Model file for the job. Use its own axes, mm. A direction names the side the tool comes from. Coordinates: 2 decimals unless noted, no trailing zeros. Write each loop counter-clockwise with the first axis right and the second up, starting at its lowest first coordinate (ties: lowest second). Pieces come first, ordered by that corner, then holes. Notation, with made-up numbers: (20, 65.25) -> (51, 65.25) arc R32 ccw to (51, 91.25) -> close; hole circle Ø1 at (16.25, 40.25). An arc over 180 degrees is marked (long way). Answer as a JSON object with one key per item and string values. Group by question number.
Autodesk Inventor part; units mm, degrees
ref_plane "YZ Plane" through (0, 0, 0) normal (1, 0, 0) x (0, 1, 0)
ref_plane "XZ Plane" through (0, 0, 0) normal (0, 1, 0) x (-1, 0, 0)
ref_plane "XY Plane" through (0, 0, 0) normal (0, 0, 1) x (1, 0, 0)
sketch "Sketch1" plane through (0, 0, 0) normal (0, 1, 0) x (-1, 0, 0)
  circle A0 centre (0, 0) radius 87.5
  dimension "d0" = 175
extrude "Plate1" add sketch "Sketch1" along normal blind 4
sketch "Sketch2" plane through (0, 4, 0) normal (0, 1, 0) x (1, 0, 0)
  circle A0 centre (0, 0) radius 87.5
  arc A1 (73.3682, -12.9368) -> (73.3682, 12.9368) centre (0, 0) ccw construction
  arc A2 (79.7694, -14.0655) -> (79.7694, 14.0655) centre (0, 0) ccw
  arc A3 (66.9669, -11.8081) -> (66.9669, 11.8081) centre (0, 0) ccw
  arc A4 (66.9669, -11.8081) -> (79.7694, -14.0655) centre (73.3682, -12.9368) ccw
  arc A5 (79.7694, 14.0655) -> (66.9669, 11.8081) centre (73.3682, 12.9368) ccw
  point P0 (74.5, 0)
  dimension "d19" = 13
  dimension "d20" = 20
  dimension "d21" = 74.5
extrude "Extrusion1" cut sketch "Sketch2" against normal through all contours A4 A3 A5 A2
pattern_circular "Circular Pattern1" count 4 over 360 about axis through (0, -10, 0) along (0, 1, 0) of "Extrusion1"
sketch "Sketch3" plane through (0, 4, 0) normal (0, 1, 0) x (1, 0, 0)
  line L0 (40.5, 40.5) -> (-40.5, 40.5)
  line L1 (-40.5, 40.5) -> (-40.5, -40.5)
  line L2 (-40.5, -40.5) -> (40.5, -40.5)
  line L3 (40.5, -40.5) -> (40.5, 40.5)
  line L4 (40.5, 40.5) -> (-40.5, -40.5) construction
  line L5 (-40.5, 40.5) -> (40.5, -40.5) construction
  point P0 (0, 0)
  dimension "d22" = 81
mark "Mark1"
equation "\"d1\" = Thickness"
equation "\"BendReliefWidth\" = Thickness"
equation "\"BendReliefDepth\" = 0.5 * Thickness"
equation "\"CornerReliefSize\" = 4 * Thickness"
equation "\"MinimumRemnant\" = 2 * Thickness"
equation "\"TransitionRadius\" = BendRadius"
equation "\"JacobiRadiusSize\" = BendRadius"
equation "\"GapSize\" = Thickness"
properties part number "MSC 906 FLANGE FRAME" material "Stainless Steel"
(1) Wall check: probe 1 along X at (y, z) = (0.25, -8); probe 2 along Z at (x, y) = (13, 1.75); probe 3 along X at (y, z) = (2.65, 7.5). Give the ranges that are in metal, low to high.
(2) Cut at D-D on x = -71. List the corners of the cut face in (y, z).
(3) Pull direction Z, two halves, no side cores. Call faces 3 (the face through (1, 0, 1)), 4 (the face through (-72.38, 2.03, 19.36)), 5 (the face through (64.49, 1.97, -59.14)): released by +Z, released by -Z, zero draft, split by the parting line, or undercut.
(4) Pin check, flat tip, straight feed: pin 1 (1.5 mm diameter, centred on x = -7.5, y = 1, fed in from -Z). Stop position of the tip, or through.
(5) 3-axis set-ups, long thin cutter, end or side, ignore diameter. For faces 1 (the face through (81, 2, 0)), 2 (the face through (1, 4, 1)): which of +Z, -Z, +X, -X, +Y, -Y reach the whole face in a straight line?
(6) Cut at B-B on x = 0. List the corners of the cut face in (y, z).
(7) Cut at A-A on z = 0. List the corners of the cut face in (x, y).
(8) Cut at C-C on y = 1.85. List the corners of the cut face in (x, z).
Results found:
{
 "1": {"probe 1": "x = -87.13 to -80.6, -67.53 to 67.53, 80.6 to 87.13", "probe 2": "z = -86.53 to -79.95, -66.87 to 66.87, 79.95 to 86.53", "probe 3": "x = -87.18 to -80.65, -67.59 to 67.59, 80.65 to 87.18"},
 "2": {"outline": "(0, -51.14) -> (4, -51.14) -> (4, -18.99) -> (0, -18.99) -> close; (0, 18.99) -> (4, 18.99) -> (4, 51.14) -> (0, 51.14) -> close"},
 "3": {"face 3": "zero draft", "face 4": "undercut", "face 5": "split by the parting line"},
 "4": {"pin 1": "stops at z = -87.24"},
 "5": {"face 1": "+Y, -Y", "face 2": "+Z, -Z, +X, -X, +Y"},
 "6": {"outline": "(0, -87.5) -> (4, -87.5) -> (4, -81) -> (0, -81) -> close; (0, -68) -> (4, -68) -> (4, 68) -> (0, 68) -> close; (0, 81) -> (4, 81) -> (4, 87.5) -> (0, 87.5) -> close"},
 "7": {"outline": "(-87.5, 0) -> (-81, 0) -> (-81, 4) -> (-87.5, 4) -> close; (-68, 0) -> (68, 0) -> (68, 4) -> (-68, 4) -> close; (81, 0) -> (87.5, 0) -> (87.5, 4) -> (81, 4) -> close"},
 "8": {"outline": "circle Ø175 at (0, 0); hole (-79.77, -14.07) arc R6.5 ccw to (-66.97, -11.81) arc R68 cw to (-66.97, 11.81) arc R6.5 ccw to (-79.77, 14.07) arc R81 ccw to start; hole (-14.07, -79.77) arc R81 ccw to (14.07, -79.77) arc R6.5 ccw to (11.81, -66.97) arc R68 cw to (-11.81, -66.97) arc R6.5 ccw to start; hole (-14.07, 79.77) arc R6.5 ccw to (-11.81, 66.97) arc R68 cw to (11.81, 66.97) arc R6.5 ccw to (14.07, 79.77) arc R81 ccw to start; hole (66.97, -11.81) arc R6.5 ccw to (79.77, -14.07) arc R81 ccw to (79.77, 14.07) arc R6.5 ccw to (66.97, 11.81) arc R68 cw to start"}
}
